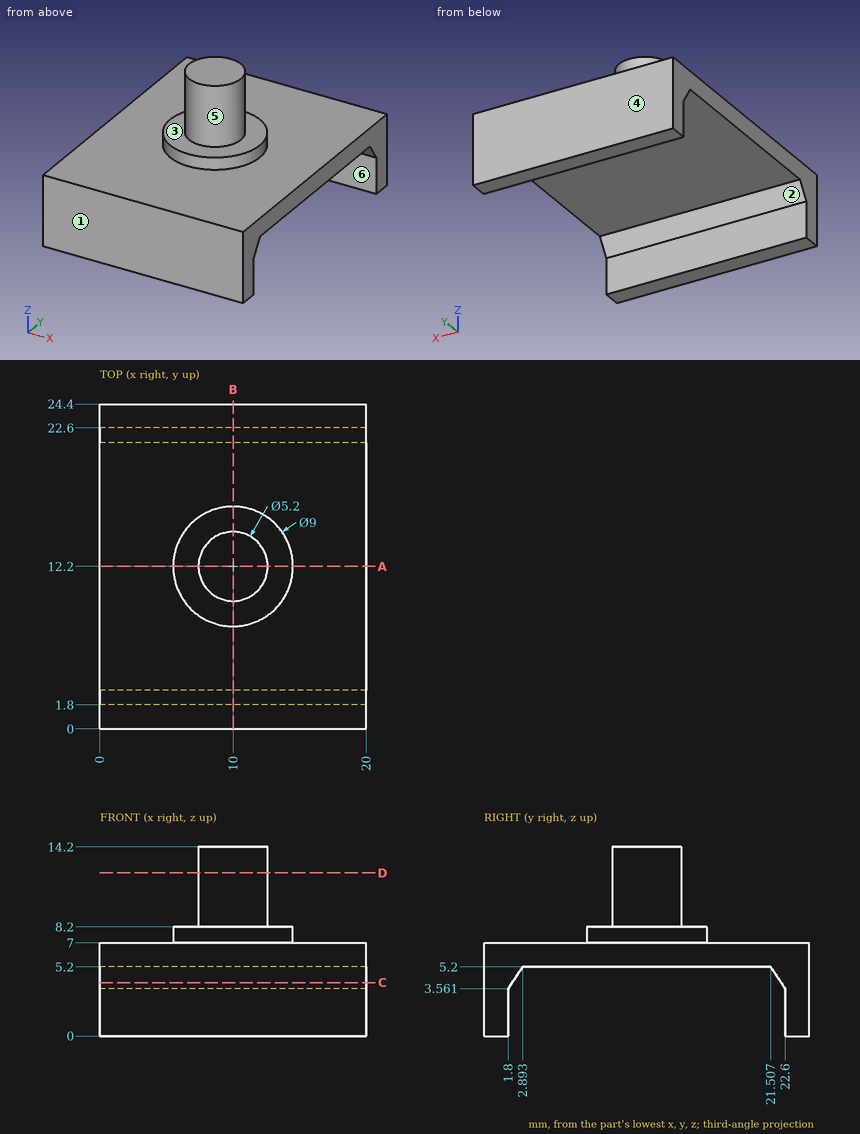
Study the drawing (mm; zero at the part's minimum x, y, z) and answer. A direction names the side the tool comes from. Round coordinates to 2 decimals unless told otherwise and drop trailing zeros. Loops run counter-clockwise (first coordinate to the right, second up) from the corner with the lowest first, then second, coordinate; pieces in that order, holes last. Notation, with made-up numbers: M 12.25,61 L 45.25,61 A30 cw 45.25,99 Z; hole C -14.75,84 d10. An arc over 180 degrees is marked long. One line per question, with ' | ' between items.
Q1. Consider line 1 along Y through (x, z) = (2, 2.5); line 2 along Z through (x, y) = (13.75, 13); line 3 along Z through (x, y) = (11, 3.25). Determine where each line is inside the solid, lowest interval first. Write a range as from..to.
Conclusion:
line 1: y = 0..1.8, 22.6..24.4 | line 2: z = 5.2..8.2 | line 3: z = 5.2..7
Q2. Find section B-B, the plane x = 10. Give the vertices of the cut face in (y, z).
Conclusion:
outline: M 0,0 L 1.8,0 L 1.8,3.56 L 2.89,5.2 L 21.51,5.2 L 22.6,3.56 L 22.6,0 L 24.4,0 L 24.4,7 L 16.7,7 L 16.7,8.2 L 14.8,8.2 L 14.8,14.2 L 9.6,14.2 L 9.6,8.2 L 7.7,8.2 L 7.7,7 L 0,7 Z
Q3. Find section C-C, the plane z = 4. Give the vertices of the cut face in (x, y).
Conclusion:
outline: M 0,0 L 20,0 L 20,2.09 L 0,2.09 Z; M 0,22.31 L 20,22.31 L 20,24.4 L 0,24.4 Z
Q4. A tool of negligible diameter and unlimited length cuts with its end or side. For the marked faces 4, 5 and 6, from which of +Z, -Z, +X, -X, +Y, -Y can it reach the whole face along a straight path? Write none if from no direction.
Conclusion:
face 4: +Z, -Z, +X, -X, +Y | face 5: +Z | face 6: -Z, +X, -X
Q5. Each of these flat-tipped pins is pushed along its axis until it touches: pin 1 Ø1.5 at (x, z) = (13.5, 8) entering from +Y; pin 2 Ø5.5 at (x, y) = (11, 13) entering from -Z. Where does it stop, or does it pass through?
Conclusion:
pin 1: stops at y = 15.76 | pin 2: stops at z = 5.2
Q6. Find section D-D, the plane z = 12.25. Give the vertices of the cut face in (x, y).
Conclusion:
outline: C 10,12.2 d5.2
Q7. The mould has two halves that part along Y. Classify the marked faces 1, 2 and 3: +Y half, -Y half, draft (parallel to the pull), parting line (faces both ways), or undercut.
Conclusion:
face 1: -Y half | face 2: undercut | face 3: draft
Q8. Find section A-A, the plane y = 12.2. Give the vertices of the cut face in (x, z).
Conclusion:
outline: M 0,5.2 L 20,5.2 L 20,7 L 14.5,7 L 14.5,8.2 L 12.6,8.2 L 12.6,14.2 L 7.4,14.2 L 7.4,8.2 L 5.5,8.2 L 5.5,7 L 0,7 Z
